Part model, mm, in its own coordinate system. Face numbers are marked on the shaded views. A direction names the side the tool comes from. Give positions to 0.01 mm unless a question says otherwise; leave off trailing zeros. Write each loop counter-clockwise with the first axis right and the second up, starting at its lowest first coordinate (ties: lowest second). Pieces come first, ordered by that corner, then holes. Notation, with made-up numbers: M 77.25,78.5 L 106.25,78.5 A22 cw 106.25,95.5 Z; hole C 18.5,63 d4. An arc over 180 degrees is marked long. Write item = value, one per line. Start each with the question number.
from build123d import *

# Parameters (mm, degrees)
SKETCH1_W           = 40
SKETCH1_H           = 40
BOSS_EXTRUDE1_DEPTH = 5.6
SKETCH2_R           = 16.925
SKETCH2_R_2         = 9.125
BOSS_EXTRUDE2_DEPTH = 54
SKETCH3_R           = 1.475
CUT_EXTRUDE1_DEPTH  = 10
FILLET1_R           = 1
CHAMFER1_SIZE       = 1.5
CUT_EXTRUDE2_START  = -10
SKETCH4_R           = 9.125
CUT_EXTRUDE2_DEPTH  = 10
SKETCH5_R           = 16.925
SKETCH5_R_2         = 6.675
BOSS_EXTRUDE3_DEPTH = 4


with BuildPart() as part:
    # Sketch1 → Boss-Extrude1 (new body)
    with BuildSketch(Plane(origin=(0, 0, 0), x_dir=(1, 0, 0), z_dir=(0, 1, 0))):
        Rectangle(SKETCH1_W, SKETCH1_H)
    extrude(amount=BOSS_EXTRUDE1_DEPTH)

    # Sketch2 → Boss-Extrude2 (add)
    with BuildSketch(Plane(origin=(0, 5.6, 0), x_dir=(1, 0, 0), z_dir=(0, 1, 0))):
        with Locations(Location((0, 0, 0), (0, 0, 270))):
            Circle(SKETCH2_R)
        with Locations(Location((0, 0, 0), (0, 0, 270))):
            Circle(SKETCH2_R_2, mode=Mode.SUBTRACT)
    extrude(amount=BOSS_EXTRUDE2_DEPTH)

    # Sketch3 → Cut-Extrude1 (cut)
    with BuildSketch(Plane.XZ):
        with Locations(Location((-16.5, -16.5, 0), (0, 0, 270))):
            Circle(SKETCH3_R)
        with Locations(Location((-16.5, 16.5, 0), (0, 0, 270))):
            Circle(SKETCH3_R)
        with Locations(Location((16.5, 16.5, 0), (0, 0, 270))):
            Circle(SKETCH3_R)
        with Locations(Location((16.5, -16.5, 0), (0, 0, 270))):
            Circle(SKETCH3_R)
    extrude(amount=-CUT_EXTRUDE1_DEPTH, mode=Mode.SUBTRACT)

    # Fillet1
    fillet1_edges = [part.edges().sort_by_distance(p)[0] for p in [
        (20, 2.8, 20),
        (-20, 2.8, 20),
        (-20, 2.8, -20),
        (20, 2.8, -20),
    ]]
    fillet(fillet1_edges, radius=FILLET1_R)

    # Chamfer1
    chamfer1_edges = [part.edges().sort_by_distance(p)[0] for p in [
        (0, 5.6, -16.925),
    ]]
    chamfer(chamfer1_edges, length=CHAMFER1_SIZE)

    # Sketch4 → Cut-Extrude2 (cut)
    with BuildSketch(Plane(origin=(0, 5.6, 0), x_dir=(1, 0, 0), z_dir=(0, 1, 0)).offset(CUT_EXTRUDE2_START)):
        with Locations(Location((0, 0, 0), (0, 0, 270))):
            Circle(SKETCH4_R)
    extrude(amount=CUT_EXTRUDE2_DEPTH, mode=Mode.SUBTRACT)

    # Sketch5 → Boss-Extrude3 (add)
    with BuildSketch(Plane(origin=(0, 59.6, 0), x_dir=(1, 0, 0), z_dir=(0, 1, 0))):
        with Locations(Location((0, 0, 0), (0, 0, 270))):
            Circle(SKETCH5_R)
        with Locations(Location((0, 0, 0), (0, 0, 270))):
            Circle(SKETCH5_R_2, mode=Mode.SUBTRACT)
    extrude(amount=BOSS_EXTRUDE3_DEPTH)


solid = part.part
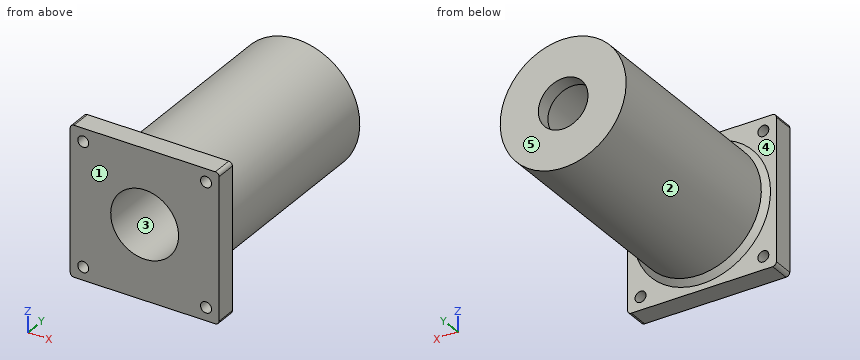
Q1. Probe line 1 along Z through (x, y) = (0, 4) (3 decimals); line 2 along Z through (x, y) = (16, 3); line 3 along X through (y, z) = (1.65, -16.5) (3 decimals). List the from-to ranges inside material, lowest first.
Q2. Tool access for the marked faces 4 and 5: list every direction of +Z, -Z, +X, -X, +Y, -Y with a clear straight run to the whole face (end or side of a thin tool).
Q3. Slice it at A-A (z = 0). Give the cut face in (x, y) (3 decimals).
Q4. Slice it at C-C (y = 23). Give the cut face in (x, z) (3 decimals), and give its area (3 significant figures).
Q5. Two-plate mould, pull along Z, no slides. Class the marked faces 1, 2 and 3: +Z half, -Z half, draft (parallel to the pull), parting line (faces both ways), or undercut.
Q6. Drop flat-ended pins along their axis: P1, Ø10, axis at x = -4, y = 40.5, coming from the +Z side (3 decimals); P2, Ø3.5, axis at x = 16.5, z = 16.5, coming from the +Y side; P3, Ø1.5, axis at y = 20.5, z = 6.5, coming from the -X side. Give the stop position or say it passes through.
Q7. Slice it at B-B (x = 0). Give the cut face in (y, z) (3 decimals).
Working result:
q1.line_1 = -20 to -9.125, 9.125 to 20
q1.line_2 = -20 to -17.89, -15.11 to 15.11, 17.89 to 20
q1.line_3 = -20 to -17.975, -15.025 to 15.025, 17.975 to 20
q2.face_4 = +Y
q2.face_5 = +Z, -Z, +X, -X, +Y
q3.outline = M -20,0 L -9.125,0 L -9.125,59.6 L -6.675,59.6 L -6.675,63.6 L -16.925,63.6 L -16.925,7.1 L -18.425,5.6 L -20,5.6 Z; M 6.675,59.6 L 9.125,59.6 L 9.125,0 L 20,0 L 20,5.6 L 18.425,5.6 L 16.925,7.1 L 16.925,63.6 L 6.675,63.6 Z
q4.outline = C 0,0 d33.85; hole C 0,0 d18.25
q4.area = 638 mm2
q5.face_1 = draft
q5.face_2 = parting line
q5.face_3 = undercut
q6.P1 = 16.925
q6.P2 = 5.6
q6.P3 = -15.92
q7.outline = M 0,-20 L 5.6,-20 L 5.6,-18.425 L 7.1,-16.925 L 63.6,-16.925 L 63.6,-6.675 L 59.6,-6.675 L 59.6,-9.125 L 0,-9.125 Z; M 0,9.125 L 59.6,9.125 L 59.6,6.675 L 63.6,6.675 L 63.6,16.925 L 7.1,16.925 L 5.6,18.425 L 5.6,20 L 0,20 Z
